Design review of the part built by this model. Coordinates are the model's own, in mm. A direction names the side the tool comes from. Coordinates: 2 decimals unless noted, no trailing zeros. Write each loop counter-clockwise with the first axis right and the second up, starting at its lowest first coordinate (ties: lowest second). Pieces come first, ordered by that corner, then holes. Notation, with made-up numbers: (11.25, 23) - (57.25, 23) arc R28 ccw to (57.25, 54) - close; hole circle Ø6 at (-15, 0.25). An arc over 180 degrees is marked (long way). Answer as a JSON object with one key per item and string values.
Autodesk Inventor part; units mm, degrees
ref_plane "YZ Plane" through (0, 0, 0) normal (1, 0, 0) x (0, 1, 0)
ref_plane "XZ Plane" through (0, 0, 0) normal (0, 1, 0) x (-1, 0, 0)
ref_plane "XY Plane" through (0, 0, 0) normal (0, 0, 1) x (1, 0, 0)
sketch "Sketch1" plane through (0, 0, 0) normal (0, 0, 1) x (1, 0, 0)
  line L0 (0, 0) -> (0, 17.4353) construction
  line L1 (0, 17.4353) -> (-3.9816, 17.4353)
  line L2 (-3.9816, 17.4353) -> (-3.9816, 16.9353)
  line L3 (-3.9816, 16.9353) -> (-2.5, 0)
  line L4 (-2.5, 0) -> (0, 0)
  line L5 (0, 17.4353) -> (3.9816, 17.4353)
  line L6 (3.9816, 17.4353) -> (3.9816, 16.9353)
  line L7 (3.9816, 16.9353) -> (2.5, 0)
  line L8 (2.5, 0) -> (0, 0)
  line L9 (-2.3884, 16.4353) -> (1.8987, 16.4353)
  line L10 (1.8987, 16.4353) -> (2.3884, 16.4353)
  line L11 (2.8865, 15.8917) -> (1.794, 3.4039)
  line L12 (-1.794, 3.4039) -> (-2.8865, 15.8917)
  arc A0 (-2.3884, 16.4353) -> (-2.8865, 15.8917) centre (-2.3884, 15.9353) ccw
  arc A1 (2.8865, 15.8917) -> (2.3884, 16.4353) centre (2.3884, 15.9353) ccw
  arc A2 (-1.794, 3.4039) -> (1.794, 3.4039) centre (0, 3.5609) ccw
  point P0 (-2.9341, 16.4353)
  point P1 (2.9341, 16.4353)
  point P2 (0, -17.1014)
  point P3 (1.8884, 16.4353)
  dimension "d1" = 5
  dimension "d2" = 0.5
  dimension "d3" = 17
  dimension "d4" = 1
  dimension "d7" = 0.5
  dimension "d8" = 5
extrude "Extrusion1" add sketch "Sketch1" along normal blind 8
properties part number "MainBracketY"
(1) The part is to be moulded in two halves that separate along Y. For faces 1 (the face through (-3, 11, 0)), 2 (the face through (0, 0, 4)), 3 (the face through (0.04, 1.76, 3.94)), say which applies: pulls with the +Y half, pulls with the -Y half, needs draft (parallel to the pull), parting line crosses it, or undercut.
Solved:
{"face 1": "needs draft", "face 2": "pulls with the -Y half", "face 3": "undercut"}
(2) Take a section at A-A, the plane z = 4.25. Write out the cut boundary in (x, y).
Solved:
{"outline": "(-3.98, 16.94) - (-2.5, 0) - (2.5, 0) - (3.98, 16.94) - (3.98, 17.44) - (-3.98, 17.44) - close; hole (-2.89, 15.89) - (-1.79, 3.4) arc R1.8 ccw to (1.79, 3.4) - (2.89, 15.89) arc R0.5 ccw to (2.39, 16.44) - (-2.39, 16.44) arc R0.5 ccw to start"}
(3) Take a section at C-C, the plane y = 7.25. Write out the cut boundary in (x, z).
Solved:
{"outline": "(-3.13, 0) - (-2.13, 0) - (-2.13, 8) - (-3.13, 8) - close; (2.13, 0) - (3.13, 0) - (3.13, 8) - (2.13, 8) - close"}
(4) Take a section at B-B, the plane x = 0.75. Write out the cut boundary in (y, z), and give its area (3 significant figures).
Solved:
{"outline": "(0, 0) - (1.92, 0) - (1.92, 8) - (0, 8) - close; (16.44, 0) - (17.44, 0) - (17.44, 8) - (16.44, 8) - close", "area": "23.4 mm^2"}
(5) Tool access review of faces 4 (the face through (-3.25, 8.59, 3.94)), 5 (the face through (2.35, 9.74, 3.94)): name each direction out of +Z, -Z, +X, -X, +Y, -Y from which nothing blocks a thin tool from reaching the whole face with its end or side.
Solved:
{"face 4": "+Z, -Z, -X, -Y", "face 5": "+Z, -Z"}
(6) To check wall thickness, follow line 1 (Y direction, x = 0, z = 2.5); line 2 (X direction, y = 15.5, z = 3.5); line 3 (X direction, y = 2.75, z = 6). State the ranges of each line that lie inside material, in increasing order. Write a range as from..to.
Solved:
{"line 1": "y = 0..1.76, 16.44..17.44", "line 2": "x = -3.86..-2.85, 2.85..3.86", "line 3": "x = -2.74..-1.61, 1.61..2.74"}
(7) Take a section at D-D, the plane x = 3.5. Write out the cut boundary in (y, z).
Solved:
{"outline": "(11.43, 0) - (17.44, 0) - (17.44, 8) - (11.43, 8) - close"}
